from build123d import *

# Parameters (mm, degrees)
SKETCH_1_W          = 36
SKETCH_1_H          = 36
SKETCH_1_R          = 2.25
EXTRUDE_1_DEPTH     = 3
SKETCH_2_W          = 36
SKETCH_2_H          = 36
EXTRUDE_2_DEPTH     = 2
SKETCH_4_R          = 9.25
CUT_EXTRUDE_1_DEPTH = 50.492465658


with BuildPart() as part:
    # 스케치1 → 보스-돌출1 (new body)
    with BuildSketch(Plane.XY):
        with Locations((17.845923561, -15.757575758)):
            Rectangle(SKETCH_1_W, SKETCH_1_H)
        with Locations((2.595923561, -0.507575758)):
            Circle(SKETCH_1_R, mode=Mode.SUBTRACT)
        with Locations((17.845923561, -0.507575758)):
            Circle(SKETCH_1_R, mode=Mode.SUBTRACT)
        with Locations((33.095923561, -0.507575758)):
            Circle(SKETCH_1_R, mode=Mode.SUBTRACT)
        with Locations((33.095923561, -15.757575758)):
            Circle(SKETCH_1_R, mode=Mode.SUBTRACT)
        with Locations((33.095923561, -31.007575758)):
            Circle(SKETCH_1_R, mode=Mode.SUBTRACT)
        with Locations((17.845923561, -31.007575758)):
            Circle(SKETCH_1_R, mode=Mode.SUBTRACT)
        with Locations((2.595923561, -31.007575758)):
            Circle(SKETCH_1_R, mode=Mode.SUBTRACT)
        with Locations((2.595923561, -15.757575758)):
            Circle(SKETCH_1_R, mode=Mode.SUBTRACT)
    extrude(amount=EXTRUDE_1_DEPTH)

    # 스케치2 → 보스-돌출2 (add)
    with BuildSketch(Plane.XY.offset(3)):
        with Locations((17.845923561, -15.757575758)):
            Rectangle(SKETCH_2_W, SKETCH_2_H)
    extrude(amount=EXTRUDE_2_DEPTH)

    # 스케치4 → 컷-돌출1 (cut, through all)
    with BuildSketch(Plane(origin=(0, 0, 0), x_dir=(-1, 0, 0), z_dir=(0, 0, -1))):
        with Locations((-17.845923561, -15.757575758)):
            Circle(SKETCH_4_R)
    extrude(amount=-CUT_EXTRUDE_1_DEPTH, mode=Mode.SUBTRACT)


solid = part.part
CAD build for the part. Positions are in the model's coordinates, mm. A direction names the side the tool comes from. Give positions to 0.01 mm unless a question says otherwise; leave off trailing zeros. Loops run counter-clockwise (first coordinate to the right, second up) from the corner with the lowest first, then second, coordinate; pieces in that order, holes last. Notation, with made-up numbers: M 8.25,23 L 61.25,23 A22 cw 61.25,37 Z; hole C 66,7.25 d5. An arc over 180 degrees is marked long. Answer in a Markdown table with one row per item. Add a question column.
Item 1: Band-saw the part on A-A on y = -10. Give the cut face in (x, z), then the cut area to 3 significant figures.
Item 2: Probe probe 1 along Y at (x, z) = (17, 1); probe 2 along X at (y, z) = (0.5, 2.95); probe 3 along Y at (x, z) = (25.5, 3.15). List the from-to ranges inside material, lowest first.
Item 3: Tool access for faces 4 (the face through (-0.154, -16, 2)), 5 (the face through (18, 0, 3)): list every direction of +Z, -Z, +X, -X, +Y, -Y with a clear straight run to the whole face (end or side of a thin tool).
Item 4: Band-saw the part on B-B on x = 10.5. Give the cut face in (y, z).
Item 5: Band-saw the part on C-C on z = 4.25. Give the cut face in (x, y).
Item 6: Band-saw the part on D-D on x = 4. Give the cut face in (y, z), then the cut area to 3 significant figures.
Item 7: Drop a flat-ended pin along its axis: P1, Ø4, axis at x = 33.1, y = -31.01, coming from the -Z side. Give the stop position or say it passes through.
Item 8: Mould opens along Y. For faces 1 (the face through (32.608, -33.204, 1.479)), 2 (the face through (10, -8, 0)), 3 (the face through (18, -33.758, 2)) say: +Y half, -Y half, draft (parallel to the pull), parting line (faces both ways), or undercut.
Reply:
| question | item | result |
|---|---|---|
| 1 | outline | M -0.15,0 L 10.61,0 L 10.61,5 L -0.15,5 Z; M 25.09,0 L 35.85,0 L 35.85,5 L 25.09,5 Z |
| 1 | area | 108 mm^2 |
| 2 | probe 1 | y = -33.76 to -33.09, -28.92 to -24.97, -6.55 to -2.59, 1.58 to 2.24 |
| 2 | probe 2 | x = -0.15 to 0.58, 4.61 to 15.83, 19.86 to 31.08, 35.11 to 35.85 |
| 2 | probe 3 | y = -33.76 to -20.95, -10.56 to 2.24 |
| 3 | face 4 | +Z, -Z, -X, +Y, -Y |
| 3 | face 5 | -Z |
| 4 | outline | M -33.76,0 L -21.38,0 L -21.38,5 L -33.76,5 Z; M -10.14,0 L 2.24,0 L 2.24,5 L -10.14,5 Z |
| 5 | outline | M -0.15,-33.76 L 35.85,-33.76 L 35.85,2.24 L -0.15,2.24 Z; hole C 17.85,-15.76 d18.5 |
| 6 | outline | M -33.76,0 L -32.77,0 L -32.77,3 L -29.25,3 L -29.25,0 L -17.52,0 L -17.52,3 L -14,3 L -14,0 L -2.27,0 L -2.27,3 L 1.25,3 L 1.25,0 L 2.24,0 L 2.24,5 L -33.76,5 Z |
| 6 | area | 148 mm^2 |
| 7 | P1 | stops at z = 3 |
| 8 | face 1 | undercut |
| 8 | face 2 | draft |
| 8 | face 3 | -Y half |
